The model under review builds one solid part; all positions refer to its coordinate system, in mm. A direction names the side the tool comes from. Coordinates: 2 decimals unless noted, no trailing zeros. Write each loop counter-clockwise with the first axis right and the second up, starting at its lowest first coordinate (ties: lowest second). Pieces come first, ordered by that corner, then holes. Notation, with made-up numbers: (57.25, -10.5) -> (77.25, -10.5) arc R31 ccw to (77.25, 18.5) -> close; hole circle Ø9 at (83, 13.5). An arc over 180 degrees is marked (long way). Put each result on its own line as item: value. Start each with the question number.
Autodesk Inventor part; units mm, degrees
ref_plane "YZ Plane" through (0, 0, 0) normal (1, 0, 0) x (0, 1, 0)
ref_plane "XZ Plane" through (0, 0, 0) normal (0, 1, 0) x (-1, 0, 0)
ref_plane "XY Plane" through (0, 0, 0) normal (0, 0, 1) x (1, 0, 0)
sketch "스케치2" plane through (0, 0, 0) normal (0, 0, 1) x (1, 0, 0)
  circle A0 centre (0, 0) radius 9
  line L0 (-3.05, -9.5235) -> (-3.05, -0.6762)
  line L1 (-3.05, -0.6762) -> (-6.7891, 7.3423)
  line L2 (3.05, 9.5235) -> (3.05, 0.6762)
  line L3 (3.05, 0.6762) -> (7.8873, -9.6974)
  line L4 (-3.05, -0.6762) -> (3.05, 0.6762) construction
  circle A1 centre (0, 0) radius 12.5
  line L5 (-11.3288, 5.2827) -> (11.3288, -5.2827)
  line L6 (8.0348, 9.5756) -> (-8.0348, -9.5756)
  circle A2 centre (0, 0) radius 10
  point P0 (5.7851, 6.8944)
  point P1 (-8.1568, 3.8036)
  point P2 (6.3427, -6.3851)
  point P3 (-5.7851, -6.8944)
  point P4 (8.1568, -3.8036)
  point P5 (-6.4279, -7.6604)
  point P6 (9.0631, -4.2262)
  point P7 (6.7891, -7.3423)
  point P8 (6.4279, 7.6604)
  point P9 (-9.0631, 4.2262)
  dimension "d12" = 18
  dimension "d14" = 6.1
  dimension "d15" = 25
  dimension "d16" = 6.1
  dimension "d17" = 25
  dimension "d19" = 40
  dimension "d20" = 40
  dimension "d36" = 20
extrude "돌출1" add sketch "스케치2" along normal blind 12.5 contours L2 L6 L5 L1 A0 | A0 L1 A2 L2 | A2 L5 A1 L6 | L2 L3 L5 L6 | L3 A2 L0 A0 | A0 L0 L6 L5 L3 | L5 A1 L3 A2 | L6 L0 L1 L5 | L3 A1 L6 A2 picked at (3.8905, 10.9384)
sketch "스케치3" plane through (0, 0, 12.5) normal (0, 0, 1) x (1, 0, 0)
  arc A0 (8.0348, 9.5756) -> (-11.3288, 5.2827) centre (0, 0) ccw
  line L0 (-11.3288, 5.2827) -> (-9.0631, 4.2262)
  line L1 (-6.7891, 7.3423) -> (-3.05, -0.6762)
  line L2 (-3.05, -0.6762) -> (-3.05, -9.5235)
  line L3 (-6.4279, -7.6604) -> (-8.0348, -9.5756)
  arc A1 (-8.0348, -9.5756) -> (11.3288, -5.2827) centre (0, 0) ccw
  line L4 (11.3288, -5.2827) -> (9.0631, -4.2262)
  line L5 (6.7891, -7.3423) -> (3.05, 0.6762)
  line L6 (3.05, 0.6762) -> (3.05, 9.5235)
  line L7 (6.4279, 7.6604) -> (8.0348, 9.5756)
  arc A2 (8.0348, 9.5756) -> (-11.3288, 5.2827) centre (0, 0) ccw
  line L8 (-2.7055, 12.2037) -> (2.7055, -12.2037)
  arc A3 (-8.0348, -9.5756) -> (11.3288, -5.2827) centre (0, 0) ccw
  line L9 (3.05, 0.6762) -> (3.05, 9.5235)
  line L10 (-3.05, -0.6762) -> (3.05, 0.6762)
  line L11 (-3.5229, 4.3404) -> (-4.6051, 9.2219)
  line L12 (-4.6051, 9.2219) -> (-6.2966, 8.8469)
  line L13 (-6.2966, 8.8469) -> (-5.2144, 3.9654)
  line L14 (-5.2144, 3.9654) -> (-3.5229, 4.3404)
  line L15 (-3.5229, 4.3404) -> (-6.2966, 8.8469) construction
  line L16 (-4.6051, 9.2219) -> (-5.2144, 3.9654) construction
  line L17 (1.3585, 5.4226) -> (0.2763, 10.3041)
  line L18 (0.2763, 10.3041) -> (1.9678, 10.679)
  line L19 (1.9678, 10.679) -> (3.05, 5.7976)
  line L20 (3.05, 5.7976) -> (1.3585, 5.4226)
  line L21 (1.3585, 5.4226) -> (1.9678, 10.679) construction
  line L22 (0.2763, 10.3041) -> (3.05, 5.7976) construction
  line L23 (-1.3585, -5.4226) -> (-0.2763, -10.3041)
  line L24 (-0.2763, -10.3041) -> (-1.9678, -10.679)
  line L25 (-1.9678, -10.679) -> (-3.05, -5.7976)
  line L26 (-3.05, -5.7976) -> (-1.3585, -5.4226)
  line L27 (-1.3585, -5.4226) -> (-1.9678, -10.679) construction
  line L28 (-0.2763, -10.3041) -> (-3.05, -5.7976) construction
  line L29 (3.5229, -4.3404) -> (4.6051, -9.2219)
  line L30 (4.6051, -9.2219) -> (5.2144, -3.9654) construction
  line L31 (4.6051, -9.2219) -> (6.2966, -8.8469)
  line L32 (6.2966, -8.8469) -> (5.2144, -3.9654)
  line L33 (5.2144, -3.9654) -> (3.5229, -4.3404)
  line L34 (3.5229, -4.3404) -> (6.2966, -8.8469) construction
  arc A4 (-6.7891, 7.3423) -> (-9.0631, 4.2262) centre (0, 0) ccw
  arc A5 (-6.4279, -7.6604) -> (-3.05, -9.5235) centre (0, 0) ccw
  arc A6 (6.7891, -7.3423) -> (9.0631, -4.2262) centre (0, 0) ccw
  arc A7 (6.4279, 7.6604) -> (3.05, 9.5235) centre (0, 0) ccw
  point P0 (3.05, 8.4674)
  point P1 (-4.9098, 6.5936)
  point P2 (1.6632, 8.0508)
  point P3 (-1.6632, -8.0508)
  point P4 (4.9098, -6.5936)
  dimension "d32" = 2.5
  dimension "d33" = 5
  dimension "d35" = 5
extrude "돌출2" add sketch "스케치3" along normal blind 15 contours L20 L17 L18 L19 | L13 L12 L11 L14 | L32 L31 L29 L33 | L26 L23 L24 L25
sketch "스케치4" plane through (0, 0, 12.5) normal (0, 0, 1) x (1, 0, 0)
  line L0 (0.2648, -12.7448) -> (-5.1462, 11.6626)
  line L1 (-5.1462, 11.6626) -> (-0.2648, 12.7448)
  line L2 (-0.2648, 12.7448) -> (5.1462, -11.6626)
  line L3 (5.1462, -11.6626) -> (0.2648, -12.7448)
  line L4 (0.2648, -12.7448) -> (-0.2648, 12.7448) construction
  line L5 (-5.1462, 11.6626) -> (5.1462, -11.6626) construction
  line L6 (-5.0577, 22.8136) -> (5.0577, -22.8136)
  circle A0 centre (0, 0) radius 3.5
  line L7 (-6.4279, -7.6604) -> (-8.0348, -9.5756)
  arc A1 (-8.0348, -9.5756) -> (11.3288, -5.2827) centre (0, 0) ccw
  line L8 (11.3288, -5.2827) -> (9.0631, -4.2262)
  arc A2 (6.7891, -7.3423) -> (9.0631, -4.2262) centre (0, 0) ccw
  line L9 (6.7891, -7.3423) -> (5.2144, -3.9654)
  line L10 (5.2144, -3.9654) -> (6.2966, -8.8469)
  line L11 (6.2966, -8.8469) -> (4.6051, -9.2219)
  line L12 (4.6051, -9.2219) -> (3.5229, -4.3404)
  line L13 (3.5229, -4.3404) -> (5.2144, -3.9654)
  line L14 (5.2144, -3.9654) -> (3.05, 0.6762)
  line L15 (3.05, 0.6762) -> (3.05, 5.7976)
  line L16 (3.05, 5.7976) -> (1.3585, 5.4226)
  line L17 (1.3585, 5.4226) -> (0.2763, 10.3041)
  line L18 (0.2763, 10.3041) -> (1.9678, 10.679)
  line L19 (1.9678, 10.679) -> (3.05, 5.7976)
  line L20 (3.05, 5.7976) -> (3.05, 9.5235)
  arc A3 (6.4279, 7.6604) -> (3.05, 9.5235) centre (0, 0) ccw
  line L21 (6.4279, 7.6604) -> (8.0348, 9.5756)
  arc A4 (8.0348, 9.5756) -> (-11.3288, 5.2827) centre (0, 0) ccw
  line L22 (-11.3288, 5.2827) -> (-9.0631, 4.2262)
  arc A5 (-6.7891, 7.3423) -> (-9.0631, 4.2262) centre (0, 0) ccw
  line L23 (-6.7891, 7.3423) -> (-5.2144, 3.9654)
  line L24 (-5.2144, 3.9654) -> (-6.2966, 8.8469)
  line L25 (-6.2966, 8.8469) -> (-4.6051, 9.2219)
  line L26 (-4.6051, 9.2219) -> (-3.5229, 4.3404)
  line L27 (-3.5229, 4.3404) -> (-5.2144, 3.9654)
  line L28 (-5.2144, 3.9654) -> (-3.05, -0.6762)
  line L29 (-3.05, -0.6762) -> (-3.05, -5.7976)
  line L30 (-3.05, -5.7976) -> (-1.3585, -5.4226)
  line L31 (-1.3585, -5.4226) -> (-0.2763, -10.3041)
  line L32 (-0.2763, -10.3041) -> (-1.9678, -10.679)
  line L33 (-1.9678, -10.679) -> (-3.05, -5.7976)
  line L34 (-3.05, -5.7976) -> (-3.05, -9.5235)
  arc A6 (-6.4279, -7.6604) -> (-3.05, -9.5235) centre (0, 0) ccw
  line L35 (-1.3585, -5.4226) -> (-3.05, -5.7976)
  line L36 (-3.05, -5.7976) -> (-1.9678, -10.679)
  line L37 (-1.9678, -10.679) -> (-0.2763, -10.3041)
  line L38 (-0.2763, -10.3041) -> (-1.3585, -5.4226)
  line L39 (6.2966, -8.8469) -> (5.2144, -3.9654)
  line L40 (5.2144, -3.9654) -> (3.5229, -4.3404)
  line L41 (3.5229, -4.3404) -> (4.6051, -9.2219)
  line L42 (4.6051, -9.2219) -> (6.2966, -8.8469)
  point P0 (1.9106, 2.9325)
  point P1 (2.9709, -1.8503)
  point P2 (-2.9709, 1.8503)
  point P3 (-1.9106, -2.9325)
  dimension "d37" = 7
extrude "돌출3" cut sketch "스케치4" against normal blind 5 contours L0 A0 L6 A1 | A1 L3 L0 | A0 L29 L28 L0 | L0 A0 L6 | A1 L2 L3 | L6 A0 L2 A1 | L0 A4 L6 A0 | A0 L28 L29 | L6 A0 L2 | L6 A4 L2 A0 | L2 A0 L15 L14 | A4 L0 L1 | L1 L2 A4 | L14 L15 A0
properties part number "_3D 인쇄"
1. Consider section D-D on z = 6.5. State the section outline as (x, y) points.
2. The part is to be moulded in two halves that separate along X. For faces 1 (the flat face through (10.18, -4.747, 6.162)), 2 (the flat face through (-2, -8, 27.5)), 3 (the cylindrical face through (4.806, 8.77, 6.162)), say which applies: released by +X, released by -X, zero draft, split by the parting line, or undercut.
3. Insertion check: P1, Ø2, axis at x = 4, y = 10.5, coming from the +Z side; P2, Ø2.5, axis at y = 3, z = 7.5, coming from the +X side; P3, Ø6, axis at y = 7, z = 8, coming from the -X side; P4, Ø3, axis at x = -3, y = -4.5, coming from the -Z side. Each pin has a flat end and moves straight along its axis. Give the tip position at first contact, or say it passes through.
4. Wall thickness on line 1 (X direction, y = 5.5, z = 10); line 2 (Z direction, x = 0.25, y = -10.5); line 3 (Y direction, x = 6.75, z = 3.5): over which ranges is each line inside the solid? List them lowest first. Write a range as from..to.
5. Consider section B-B on y = 6.75. State the section outline as (x, z) points.
6. Consider section C-C on x = -4.25. State the section outline as (y, z) points, then the cut area to 3 significant figures.
7. Consider section A-A on z = 16.25. State the section outline as (x, y) points, then the cut area to 3 significant figures.
8. Tool access review of faces 4 (the flat face through (-5.763, 6.44, 19.895)), 5 (the flat face through (-2.216, -5.613, 19.895)), 6 (the flat face through (5.763, -6.44, 19.895)), 7 (the flat face through (-4.38, 4.15, 19.9)), 8 (the flat face through (-7.22, -8.605, 6.162)): name each direction out of +Z, -Z, +X, -X, +Y, -Y from which nothing blocks a thin tool from reaching the whole face with its end or side.
Output values:
1. outline: (-11.33, 5.28) -> (-9.06, 4.23) arc R10 cw to (-6.79, 7.34) -> (-3.05, -0.68) -> (-3.05, -9.52) arc R10 cw to (-6.43, -7.66) -> (-8.03, -9.58) arc R12.5 ccw to (11.33, -5.28) -> (9.06, -4.23) arc R10 cw to (6.79, -7.34) -> (3.05, 0.68) -> (3.05, 9.52) arc R10 cw to (6.43, 7.66) -> (8.03, 9.58) arc R12.5 ccw to start
2. face 1: released by +X
2. face 2: zero draft
2. face 3: undercut
3. P1: stops at z = 12.5
3. P2: stops at x = 3.05
3. P3: stops at x = -11.33
3. P4: stops at z = 0
4. line 1: x = -11.22..-8.35, -5.93..-3.78, 1.34..3.05
4. line 2: z = 0..7.5
4. line 3: y = -10.52..-7.26, 8.04..10.52
5. outline: (-10.52, 0) -> (-7.38, 0) -> (-7.38, 12.5) -> (-10.52, 12.5) -> close; (-6.51, 0) -> (3.05, 0) -> (3.05, 12.5) -> (2.84, 12.5) -> (2.84, 27.5) -> (1.06, 27.5) -> (1.06, 7.5) -> (-4.06, 7.5) -> (-4.06, 27.5) -> (-5.83, 27.5) -> (-5.83, 12.5) -> (-6.51, 12.5) -> close
6. outline: (-11.76, 0) -> (-9.05, 0) -> (-9.05, 12.5) -> (-11.76, 12.5) -> close; (1.9, 0) -> (11.76, 0) -> (11.76, 7.5) -> (7.62, 7.5) -> (7.62, 27.5) -> (4.18, 27.5) -> (4.18, 12.5) -> (1.9, 12.5) -> close
6. area: 188 mm^2
7. outline: (-6.3, 8.85) -> (-5.21, 3.97) -> (-3.52, 4.34) -> (-4.61, 9.22) -> close; (-3.05, -5.8) -> (-1.97, -10.68) -> (-0.28, -10.3) -> (-1.36, -5.42) -> close; (0.28, 10.3) -> (1.36, 5.42) -> (3.05, 5.8) -> (1.97, 10.68) -> close; (3.52, -4.34) -> (4.61, -9.22) -> (6.3, -8.85) -> (5.21, -3.97) -> close
7. area: 34.7 mm^2
8. face 4: +Z, -X, -Y
8. face 5: +Z, -X, +Y
8. face 6: +Z, +X, +Y
8. face 7: +Z, +X, -Y
8. face 8: +Z, -Z, -X
